Could you check a few things on this model? Use its own coordinates, in mm. A direction names the side the tool comes from. Give positions to 0.01 mm unless a question says otherwise; leave off trailing zeros. Loops run counter-clockwise (first coordinate to the right, second up) from the corner with the lowest first, then second, coordinate; pieces in that order, holes last. Notation, with made-up numbers: M 5,33.25 L 14,33.25 A22 cw 14,39.25 Z; hole C -24.5,81 d10. An arc over 180 degrees is marked long. Return JSON: item names as keys, results as strings. Group by question number.
1. If we section it at A-A (y = 442): Write out the boundary of the cut face in (x, z).
2. For faces 1 (the flat face through (-7, 449, 180)), 2 (the flat face through (500, 449, 145)), 3 (the flat face through (-2, 449, 120)), which set-ups out of +Z, -Z, +X, -X, +Y, -Y let a thin tool reach every point of the face, with its end or its side?
3. Please list where these lines run through material, in increasing order: line 1 (Z direction, x = -473.5, y = 460); line 2 (Y direction, x = 334, z = 261); line 3 (Y direction, x = 348.5, z = 18).
4. If we section it at B-B (x = -420): Write out the boundary of the cut face in (y, z), plus the area to 3 significant figures.
5. For pin 1 (3 mm diameter, centred on x = -115, z = 264.5, fed in from +Y); pin 2 (12 mm diameter, centred on y = 452, z = 158, fed in from -X), each with a flat end and sliding along its axis, tell me the tip position at first contact or that it passes through.
6. If we section it at C-C (z = 56): Write out the boundary of the cut face in (x, y).
```python
from build123d import *

# Parameters (mm, degrees)
SKETCH_1_W      = 1300
SKETCH_1_H      = 800
EXTRUDE_1_DEPTH = 300
FILLET_1_R      = 30
SKETCH_2_W      = 1000
SKETCH_2_H      = 60
EXTRUDE_2_DEPTH = 100
FILLET_2_R      = 10


with BuildPart() as part:
    # 草图1 → 凸台-拉伸1 (new body)
    with BuildSketch(Plane.XY):
        Rectangle(SKETCH_1_W, SKETCH_1_H)
    extrude(amount=EXTRUDE_1_DEPTH)

    # 圆角1
    fillet_1_edges = [part.edges().sort_by_distance(p)[0] for p in [
        (650, 0, 300),
        (0, 400, 300),
        (-650, 0, 300),
        (0, 400, 0),
        (650, 0, 0),
        (0, -400, 0),
        (-650, 0, 0),
        (0, -400, 300),
        (-650, 400, 150),
        (650, 400, 150),
        (650, -400, 150),
        (-650, -400, 150),
    ]]
    fillet(fillet_1_edges, radius=FILLET_1_R)

    # 草图2 → 凸台-拉伸2 (add)
    with BuildSketch(Plane(origin=(0, 400, 0), x_dir=(1, 0, 0), z_dir=(0, 1, 0))):
        with Locations((0, -150)):
            Rectangle(SKETCH_2_W, SKETCH_2_H)
    extrude(amount=EXTRUDE_2_DEPTH)

    # 圆角2
    fillet_2_edges = [part.edges().sort_by_distance(p)[0] for p in [
        (-500, 400, 150),
        (-500, 450, 120),
        (0, 400, 180),
        (-500, 450, 180),
        (500, 400, 150),
        (500, 450, 180),
        (0, 400, 120),
        (-500, 500, 150),
        (0, 500, 180),
        (500, 500, 150),
        (0, 500, 120),
    ]]
    fillet(fillet_2_edges, radius=FILLET_2_R)


solid = part.part
```
Answer:
{
 "1": {"outline": "M -500,130 A10 ccw -490,120 L 500,120 L 500,170 A10 ccw 490,180 L -490,180 A10 ccw -500,170 Z"},
 "2": {"face 1": "+Z, +X, -X, +Y", "face 2": "+Z, -Z, +X, +Y", "face 3": "-Z, +X, -X, +Y"},
 "3": {"line 1": "z = 120 to 180", "line 2": "y = -400 to 400", "line 3": "y = -397.5 to 397.5"},
 "4": {"outline": "M -400,30 A30 ccw -370,0 L 370,0 A30 ccw 400,30 L 400,110 A10 cw 410,120 L 490,120 A10 ccw 500,130 L 500,170 A10 ccw 490,180 L 410,180 A10 cw 400,190 L 400,270 A30 ccw 370,300 L -370,300 A30 ccw -400,270 Z", "area": "245,000 mm²"},
 "5": {"pin 1": "stops at y = 400", "pin 2": "stops at x = -500"},
 "6": {"outline": "M -650,-370 A30 ccw -620,-400 L 620,-400 A30 ccw 650,-370 L 650,370 A30 ccw 620,400 L -620,400 A30 ccw -650,370 Z"}
}
